Source: CAD feature listing. Evaluate the final solid. Frame: model axes, mm. A direction names the side the tool comes from. Round coordinates to 2 decimals unless told otherwise and drop trailing zeros. Loops run counter-clockwise (first coordinate to the right, second up) from the corner with the lowest first, then second, coordinate; pieces in that order, holes last. Notation, with made-up numbers: (-3, 30) - (25, 30) arc R37 cw to (25, 68) - close; hole circle Ø11 at (27, -16). An arc over 180 degrees is marked (long way). One line per question, with ' | ' between items.
Autodesk Inventor part; units mm, degrees
ref_plane "YZ Plane" through (0, 0, 0) normal (1, 0, 0) x (0, 1, 0)
ref_plane "XZ Plane" through (0, 0, 0) normal (0, 1, 0) x (-1, 0, 0)
ref_plane "XY Plane" through (0, 0, 0) normal (0, 0, 1) x (1, 0, 0)
sketch "Sketch1" plane through (0, 0, 0) normal (1, 0, 0) x (0, 1, 0)
  circle A0 centre (0, 0) radius 6.35
  line L0 (0, 0) -> (0, 6.35) construction
  line L1 (-1.5875, 6.1484) -> (-1.5875, 4.7625)
  line L2 (-1.5875, 4.7625) -> (1.5875, 4.7625)
  line L3 (1.5875, 4.7625) -> (1.5875, 6.1484)
  point P0 (0, 4.7625)
  dimension "d0" = 12.7
  dimension "d2" = 1.5875
  dimension "d3" = 3.175
extrude "Extrusion1" add sketch "Sketch1" along normal blind 76.2
sketch "Sketch2" plane through (76.2, 0, 0) normal (1, 0, 0) x (0, 0, -1)
  circle A0 centre (0, 0) radius 6.35
  circle A1 centre (0, 0) radius 4.7625
  dimension "d6" = 9.525
extrude "Extrusion2" add sketch "Sketch2" along normal blind 12.7 contours A1
extrude "Extrusion3" cut sketch "Sketch1" along normal blind 69.85 contours L3 L2 L1 A0 picked at (0.1781, 5.2842)
fillet "Fillet1" radius 1.5875 2 edges at (69.85, 1.5875, 5.4554) (69.85, -1.5875, 5.4554)
chamfer "Chamfer1" distance 1.27 distance2 2.54 1 edges at (0, 0, -6.35) measured on face at (50.8, -3.3725, 5.3804)
sketch "Sketch3" plane through (0, 0, 0) normal (-1, 0, 0) x (0, 0, 1)
  circle A0 centre (0, 0) radius 3.81
  circle A1 centre (0, 0) radius 2.3495
  dimension "d16" = 4.699
extrude "Extrusion4" cut sketch "Sketch3" against normal blind 12.7 contours A1
thread "Thread1"
properties part number "Banebots 0.5x3 P60 Shaft" material "Steel, Carbon"
1. Section query B-B, the plane z = 0. Return loops of the section in (x, y).
Worked out:
outline: (0, -3.81) - (1.27, -6.35) - (76.2, -6.35) - (76.2, -4.76) - (88.9, -4.76) - (88.9, 4.76) - (76.2, 4.76) - (76.2, 6.35) - (1.27, 6.35) - (0, 3.81) - (0, 2.35) - (12.7, 2.35) - (12.7, -2.35) - (0, -2.35) - close
2. Material intervals for probe 1 along Y at (x, z) = (3.5, 0); probe 2 along X at (y, z) = (0.25, 1.5); probe 3 along X at (y, z) = (0, -5.75), sorted ascending.
Worked out:
probe 1: y = -6.35 to -2.35, 2.35 to 6.35 | probe 2: x = 12.7 to 88.9 | probe 3: x = 0.97 to 76.2
3. Contact query for flat-ended pins moving along their axis: P1, Ø1.5, axis at x = 40, z = 2, coming from the +Y side; P2, Ø0.7, axis at x = 22.5, z = 5.5, coming from the +Y side; P3, Ø1, axis at x = 35.5, y = 0.5, coming from the +Z side. Output: stop coordinate, or through.
Worked out:
P1: stops at y = 6.23 | P2: stops at y = 3.71 | P3: stops at z = 4.76
4. Section query D-D, the plane x = 24.5. Return loops of the section in (y, z).
Worked out:
outline: (-1.59, 4.76) - (-1.59, 6.15) arc R6.35 ccw (long way) to (1.59, 6.15) - (1.59, 4.76) - close
5. Mould query, pull axis Z, two halves, no side actions, for faces 6 (the flat face through (35, 0, 4.762)), 7 (the cylindrical face through (6.26, 2.33, -0.31)), 8 (the cylindrical face through (82.46, 2.9, 3.78)), 9 (the flat face through (34, -1.588, 5)). Classes: released by +Z, released by -Z, zero draft, split by the parting line, or undercut.
Worked out:
face 6: released by +Z | face 7: undercut | face 8: split by the parting line | face 9: zero draft
6. Section query A-A, the plane y = 0. Return loops of the section in (x, z).
Worked out:
outline: (0, -3.81) - (1.27, -6.35) - (76.2, -6.35) - (76.2, -4.76) - (88.9, -4.76) - (88.9, 4.76) - (76.2, 4.76) - (76.2, 6.35) - (69.85, 6.35) - (69.85, 4.76) - (0.48, 4.76) - (0, 3.81) - (0, 2.35) - (12.7, 2.35) - (12.7, -2.35) - (0, -2.35) - close
7. Access query for faces 1 (the flat face through (88.9, 0, 0)), 2 (the flat face through (0, -2, -2)), 3 (the flat face through (76.2, 1, 5)), 4 (the flat face through (34, 1.588, 5)), 5 (the flat face through (12.7, 0, 0)). Directions: +Z, -Z, +X, -X, +Y, -Y. A direction counts if a zero-diameter tool reaches every point of the face in a straight line with its end or side. Return the directions, or none.
Worked out:
face 1: +Z, -Z, +X, +Y, -Y | face 2: +Z, -Z, -X, +Y, -Y | face 3: +X | face 4: +Z, -X | face 5: -X
8. Section query C-C, the plane x = 80. Return loops of the section in (y, z) (1 decimal), plus the area to 3 significant figures.
Worked out:
outline: circle Ø9.5 at (0, 0) | area: 71.3 mm2
